from build123d import *

# Parameters (mm, degrees)
CYLINDER_R            = 38.4
CYLINDER_DEPTH        = 2
SKETCH_R              = 1.5
POCKET_DEPTH          = 217.261029
POCKET_DEPTH_BACK     = 219.261029
POLARPATTERN_COUNT    = 3
SKETCH001_R           = 7
POCKET001_DEPTH       = 0.001
POCKET001_DEPTH_BACK  = 2.001
SKETCH002_R           = 7
POCKET002_DEPTH       = 217.261029
POCKET002_DEPTH_BACK  = 219.261029
POLARPATTERN001_COUNT = 6
SKETCH003_W           = 6
SKETCH003_H           = 3.25
POCKET003_DEPTH       = 217.261029
POCKET003_DEPTH_BACK  = 219.261029
POLARPATTERN002_COUNT = 3


with BuildPart() as part:
    # Cylinder → Cylinder (new body)
    with BuildSketch(Plane.XY):
        Circle(CYLINDER_R)
    extrude(amount=CYLINDER_DEPTH)

    # Sketch → Pocket (cut, two sides)
    with BuildSketch(Plane(origin=(34, 0, 0), x_dir=(1, 0, 0), z_dir=(0, 0, 1))) as pocket_sk:
        Circle(SKETCH_R)
    pocket = extrude(amount=-POCKET_DEPTH, mode=Mode.SUBTRACT) + extrude(pocket_sk.sketch, amount=POCKET_DEPTH_BACK, mode=Mode.SUBTRACT)

    # PolarPattern: Pocket ×3 about axis
    polarpattern_axis = Axis((0, 0, 0), (0, 0, 1))
    for i in range(1, POLARPATTERN_COUNT):
        add(pocket.rotate(polarpattern_axis, i * 360 / POLARPATTERN_COUNT), mode=Mode.SUBTRACT)

    # Sketch001 → Pocket001 (cut, two sides)
    with BuildSketch(Plane.XY) as pocket001_sk:
        Circle(SKETCH001_R)
    extrude(amount=-POCKET001_DEPTH, mode=Mode.SUBTRACT)
    extrude(pocket001_sk.sketch, amount=POCKET001_DEPTH_BACK, mode=Mode.SUBTRACT)

    # Sketch002 → Pocket002 (cut, two sides)
    with BuildSketch(Plane(origin=(0, 25, 0), x_dir=(1, 0, 0), z_dir=(0, 0, 1))) as pocket002_sk:
        Circle(SKETCH002_R)
    pocket002 = extrude(amount=-POCKET002_DEPTH, mode=Mode.SUBTRACT) + extrude(pocket002_sk.sketch, amount=POCKET002_DEPTH_BACK, mode=Mode.SUBTRACT)

    # PolarPattern001: Pocket002 ×6 about axis
    polarpattern001_axis = Axis((0, 0, 0), (0, 0, 1))
    for i in range(1, POLARPATTERN001_COUNT):
        add(pocket002.rotate(polarpattern001_axis, i * 360 / POLARPATTERN001_COUNT), mode=Mode.SUBTRACT)

    # Sketch003 → Pocket003 (cut, two sides)
    with BuildSketch(Plane(origin=(-33, 0, 0), x_dir=(1, 0, 0), z_dir=(0, 0, 1))) as pocket003_sk:
        Rectangle(SKETCH003_W, SKETCH003_H)
    pocket003 = extrude(amount=-POCKET003_DEPTH, mode=Mode.SUBTRACT) + extrude(pocket003_sk.sketch, amount=POCKET003_DEPTH_BACK, mode=Mode.SUBTRACT)

    # PolarPattern002: Pocket003 ×3 about axis
    polarpattern002_axis = Axis((0, 0, 0), (0, 0, 1))
    for i in range(1, POLARPATTERN002_COUNT):
        add(pocket003.rotate(polarpattern002_axis, i * 360 / POLARPATTERN002_COUNT), mode=Mode.SUBTRACT)


solid = part.part
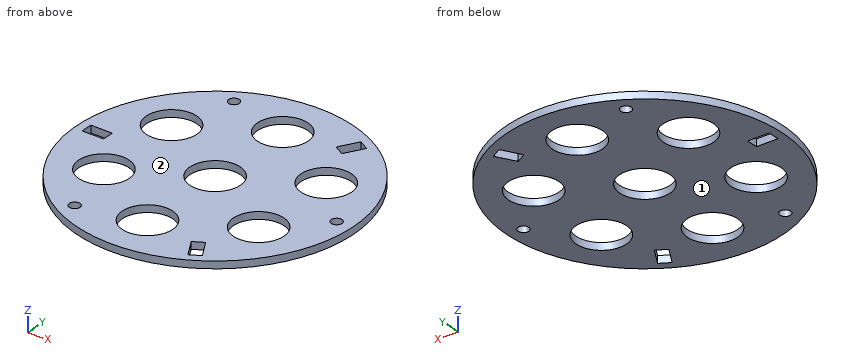
Input: part model. Units: mm. Frame: model coordinates. Face numbers are marked on the shaded views. Round coordinates to 2 decimals unless told otherwise and drop trailing zeros. Write each loop counter-clockwise with the first axis right and the second up, starting at its lowest first coordinate (ties: lowest second). Pieces come first, ordered by that corner, then holes.
1) Cut plane A-A (y = 0). Return the cut outline in (x, z).
2) Ray query, L1, parallel to Y at x = 0, z = 0.15; L2, parallel to Y at x = 14.5, z = 1.25; L3, parallel to Y at x = -4.5, z = 0.9. Return the intervals inside material, ascending.
3) Cut plane B-B (x = 0). Return the cut outline in (y, z), then the cut area to 3 significant figures.
4) Cut plane C-C (x = 34). Return the cut outline in (y, z), then the cut area to 3 significant figures.
5) Cut plane D-D (z = 1.55). Count the separate pieces of the cut face and the enclosed holes in it, then the cut area to 3 significant figures.
6) Draft query along Z for the marked faces 1 and 2. Return one class per face: pulls with the +Z half, pulls with the -Z half, needs draft (parallel to the pull), parting line crosses it, or undercut.
7) Contact query for flat-ended pins moving along their axis: P1, Ø11, axis at x = 0, y = 0, coming from the +Z side; P2, Ø1, axis at x = -13.5, z = 1.5, coming from the +Y side; P3, Ø0.6, axis at x = -33, z = 0.5, coming from the -Y side. Output: stop coordinate, or through.
Geometry says:
1. outline: (-38.4, 0) - (-36, 0) - (-36, 2) - (-38.4, 2) - close; (-30, 0) - (-7, 0) - (-7, 2) - (-30, 2) - close; (7, 0) - (32.5, 0) - (32.5, 2) - (7, 2) - close; (35.5, 0) - (38.4, 0) - (38.4, 2) - (35.5, 2) - close
2. L1: y = -38.4 to -32, -18 to -7, 7 to 18, 32 to 38.4
2. L2: y = -35.56 to -28.36, -26.27 to 26.27, 28.36 to 35.56
2. L3: y = -38.14 to -30.36, -19.64 to -5.36, 5.36 to 19.64, 30.36 to 38.14
3. outline: (-38.4, 0) - (-32, 0) - (-32, 2) - (-38.4, 2) - close; (-18, 0) - (-7, 0) - (-7, 2) - (-18, 2) - close; (7, 0) - (18, 0) - (18, 2) - (7, 2) - close; (32, 0) - (38.4, 0) - (38.4, 2) - (32, 2) - close
3. area: 69.6 mm2
4. outline: (-17.85, 0) - (-1.5, 0) - (-1.5, 2) - (-17.85, 2) - close; (1.5, 0) - (17.85, 0) - (17.85, 2) - (1.5, 2) - close
4. area: 65.4 mm2
5. separate pieces: 1
5. enclosed holes: 13
5. area: 3,480 mm2
6. face 1: pulls with the -Z half
6. face 2: pulls with the +Z half
7. P1: passes through
7. P2: stops at y = 36.13
7. P3: stops at y = -20.13
